Geometry: final body of the model. Coordinates: model frame, mm. Face numbers are marked on the shaded views. A direction names the side the tool comes from. Give positions to 0.01 mm unless a question says otherwise; leave off trailing zeros. Order: outer loops, then holes, each group sorted by start corner. A loop starts at its lowest first (then second) coordinate and runs counter-clockwise, first axis right, second up. Notation, with made-up numbers: (11, -4.5) -> (62, -4.5) arc R33 ccw to (62, 31.5) -> close; hole circle Ø4 at (89, 0). An arc over 180 degrees is marked (long way). Answer in a Markdown table with one row per item. Add a question column.
Q1. Contact query for flat-ended pins moving along their axis: P1, Ø1, axis at x = 24, z = 4.5, coming from the -Y side; P2, Ø6, axis at y = 11.5, z = -5, coming from the -X side; P3, Ø8, axis at x = 39.5, y = 12, coming from the -Z side; P4, Ø1.5, axis at y = 3.5, z = 13.5, coming from the +X side. Output: stop coordinate, or through.
Q2. Cut plane D-D on y = 0. Return the cut outline in (x, z), and give its area (3 significant figures).
Q3. Cut plane A-A on x = 3. Return the cut outline in (y, z).
Q4. Cut plane B-B on y = 12.5. Return the cut outline in (x, z).
Q5. Set-up query: the marked faces 1 and 2. Return all of +Z, -Z, +X, -X, +Y, -Y with unobstructed straight access to the full face (end or side cutting, diameter ignored); none if empty.
Q6. Line query: line 1 along Z through (x, y) = (3.8, -12.5); line 2 along X through (y, z) = (-1, -7); line 3 along Z through (x, y) = (3, 12). Output: solid intervals per line, ascending. Write a range as from..to.
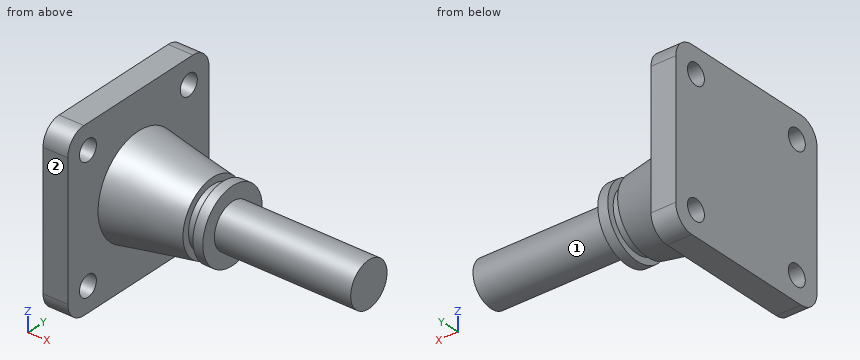
from build123d import *

# Parameters (mm, degrees)
SKETCH4_OUTSIDE_W       = 94.32
SKETCH4_OUTSIDE_H       = 94.32
SKETCH4_OUTSIDE_W_2     = 35
SKETCH4_OUTSIDE_H_2     = 35
CUT_EXTRUDE1_DEPTH      = 5
FILLET1_R               = 4
CUT_EXTRUDE2_DEPTH      = 53.697949186
CUT_EXTRUDE2_DEPTH_BACK = 53.697949186
SKETCH5_R               = 2.1


with BuildPart() as part:
    # Sketch3 → Revolve1 (revolve)
    with BuildSketch(Plane(origin=(0, 0, 0), x_dir=(1, 0, 0), z_dir=(0, 1, 0)), mode=Mode.PRIVATE) as revolve1_sk:
        Polygon((0, 0), (0, 35), (5, 35), (5, 10), (20, 7.355095289), (20, 6), (22, 6), (22, 7.355095289), (24, 7.355095289), (24, 4.5), (51.524980907, 4.5), (51.524980907, 0), align=None)
    revolve(revolve1_sk.sketch.rotate(Axis((0, 0, 0), (1, 0, 0)), 180), axis=Axis((0, 0, 0), (1, 0, 0)))

    # Sketch4 outside → Cut-Extrude1 (cut)
    with BuildSketch(Plane(origin=(5, 0, 0), x_dir=(0, 0, -1), z_dir=(1, 0, 0))):
        Rectangle(SKETCH4_OUTSIDE_W, SKETCH4_OUTSIDE_H)
        Rectangle(SKETCH4_OUTSIDE_W_2, SKETCH4_OUTSIDE_H_2, mode=Mode.SUBTRACT)
    extrude(amount=-CUT_EXTRUDE1_DEPTH, mode=Mode.SUBTRACT)

    # Fillet1
    fillet1_edges = [part.edges().sort_by_distance(p)[0] for p in [
        (2.5, -17.5, -17.5),
        (2.5, -17.5, 17.5),
        (2.5, 17.5, 17.5),
        (2.5, 17.5, -17.5),
    ]]
    fillet(fillet1_edges, radius=FILLET1_R)

    # Sketch5 → Cut-Extrude2 (cut, two sides: drawn at the far end of the back side and taken through both)
    with BuildSketch(Plane(origin=(5, 0, 0), x_dir=(0, 0, -1), z_dir=(1, 0, 0)).offset(-CUT_EXTRUDE2_DEPTH_BACK)):
        with Locations((-12.5, 12.5)):
            Circle(SKETCH5_R)
        with Locations((12.5, 12.5)):
            Circle(SKETCH5_R)
        with Locations((12.5, -12.5)):
            Circle(SKETCH5_R)
        with Locations((-12.5, -12.5)):
            Circle(SKETCH5_R)
    extrude(amount=CUT_EXTRUDE2_DEPTH + CUT_EXTRUDE2_DEPTH_BACK, mode=Mode.SUBTRACT)


solid = part.part
Completed:
| question | item | result |
|---|---|---|
| 1 | P1 | stops at y = -6.17 |
| 1 | P2 | stops at x = 0 |
| 1 | P3 | passes through |
| 1 | P4 | stops at x = 5 |
| 2 | outline | (0, -17.5) -> (5, -17.5) -> (5, -10) -> (20, -7.36) -> (20, -6) -> (22, -6) -> (22, -7.36) -> (24, -7.36) -> (24, -4.5) -> (51.52, -4.5) -> (51.52, 4.5) -> (24, 4.5) -> (24, 7.36) -> (22, 7.36) -> (22, 6) -> (20, 6) -> (20, 7.36) -> (5, 10) -> (5, 17.5) -> (0, 17.5) -> close |
| 2 | area | 736 mm² |
| 3 | outline | (-17.5, -13.5) arc R4 ccw to (-13.5, -17.5) -> (13.5, -17.5) arc R4 ccw to (17.5, -13.5) -> (17.5, 13.5) arc R4 ccw to (13.5, 17.5) -> (-13.5, 17.5) arc R4 ccw to (-17.5, 13.5) -> close; hole circle Ø4.2 at (-12.5, -12.5); hole circle Ø4.2 at (-12.5, 12.5); hole circle Ø4.2 at (12.5, -12.5); hole circle Ø4.2 at (12.5, 12.5) |
| 4 | outline | (0, -17.5) -> (5, -17.5) -> (5, -14.6) -> (0, -14.6) -> close; (0, -10.4) -> (5, -10.4) -> (5, 10.4) -> (0, 10.4) -> close; (0, 14.6) -> (5, 14.6) -> (5, 17.5) -> (0, 17.5) -> close |
| 5 | face 1 | +X |
| 5 | face 2 | +Z, -Z, +X, -X, -Y |
| 6 | line 1 | z = -17.5..-14.6, -10.4..10.4, 14.6..17.5 |
| 6 | line 2 | x = 0..20, 22..24 |
| 6 | line 3 | z = -17.5..-14.54, -10.46..10.46, 14.54..17.5 |
